Read the model definition and answer for the solid it produces. Units are mm, in the model's axes. A direction names the side the tool comes from. Round coordinates to 2 decimals unless told otherwise and drop trailing zeros. Write each loop counter-clockwise with the first axis right and the second up, starting at its lowest first coordinate (ties: lowest second). Pieces come first, ordered by that corner, then holes. Notation, with made-up numbers: (-6, 45) - (31, 45) arc R25 cw to (31, 80) - close; hole circle Ø2 at (58, 61). An arc over 180 degrees is marked (long way). Use one line per item in the form item = value. Start each with the question number.
1) For a pull along Z with two mould halves and no side action, classify faces 1 (the face through (0, 0, -85)), 2 (the face through (0, 5, 45)), 3 (the face through (-1, 16.07, 47.54)) as released by +Z, released by -Z, zero draft, split by the parting line, or undercut.
2) The part is cut by section B-B, the plane y = -2. Count the separate pieces of the cut face and the enclosed holes in it, plus the area to 3 significant figures.
3) Consider line 1 along Y through (x, z) = (1.6, 61); line 2 along Y through (x, z) = (1.4, -74.5). Determine where each line is inside the solid, lowest interval first. Write a range as from..to.
4) Each of these flat-tipped pins is pushed along its axis until it touches: pin 1 (1.5 mm diameter, centred on x = 0, z = -16.5, fed in from +Y); pin 2 (1.5 mm diameter, centred on x = -0.5, y = 8, fed in from +Z). Where does it stop, or does it pass through?
5) The part is cut by section A-A, the plane z = -29. Give the vertices of the cut face in (x, y), plus the area to 3 significant figures.
6) For faces 4 (the face through (-1, 16.07, -52.46)), 5 (the face through (0, 5, -15)), 6 (the face through (0, 5, 80)), determine the directions among +Z, -Z, +X, -X, +Y, -Y from which every point of the face is accessible in a straight line to the end or side of a thin tool.
from build123d import *

# Parameters (mm, degrees)
SALIENTE_EXTRUIR1_DEPTH = 85
CROQUIS2_W              = 5
CROQUIS2_H              = 25
CORTAR_EXTRUIR1_DEPTH   = 6
CROQUIS3_W              = 5
CROQUIS3_H              = 10
SALIENTE_EXTRUIR2_DEPTH = 45
CROQUIS4_W              = 1
CROQUIS4_H              = 25
CORTAR_EXTRUIR2_DEPTH   = 6


with BuildPart() as part:
    # Croquis1 → Saliente-Extruir1 (new body, symmetric)
    with BuildSketch(Plane.XY):
        with BuildLine():
            Line((-2.5, -17.5), (2.5, -17.5))
            Line((2.5, -17.5), (2.5, 17.5))
            ThreePointArc((2.5, 17.5), (-1.035533906, 16.035533906), (-2.5, 12.5))
            Line((-2.5, 12.5), (-2.5, -17.5))
        make_face()
    extrude(amount=SALIENTE_EXTRUIR1_DEPTH, both=True)

    # Croquis2 → Cortar-Extruir1 (cut, through all)
    with BuildSketch(Plane(origin=(2.5, 0, 0), x_dir=(0, 0, -1), z_dir=(1, 0, 0))):
        with Locations((77.5, 5)):
            Rectangle(CROQUIS2_W, CROQUIS2_H)
        with Locations((67.5, 5)):
            Rectangle(CROQUIS2_W, CROQUIS2_H)
        with Locations((57.5, 5)):
            Rectangle(CROQUIS2_W, CROQUIS2_H)
        with Locations((47.5, 5)):
            Rectangle(CROQUIS2_W, CROQUIS2_H)
        with Locations((37.5, 5)):
            Rectangle(CROQUIS2_W, CROQUIS2_H)
        with Locations((27.5, 5)):
            Rectangle(CROQUIS2_W, CROQUIS2_H)
        with Locations((17.5, 5)):
            Rectangle(CROQUIS2_W, CROQUIS2_H)
        with Locations((7.5, 5)):
            Rectangle(CROQUIS2_W, CROQUIS2_H)
        with Locations((-2.5, 5)):
            Rectangle(CROQUIS2_W, CROQUIS2_H)
        with Locations((-12.5, 5)):
            Rectangle(CROQUIS2_W, CROQUIS2_H)
        with Locations((-22.5, 5)):
            Rectangle(CROQUIS2_W, CROQUIS2_H)
        with Locations((-32.5, 5)):
            Rectangle(CROQUIS2_W, CROQUIS2_H)
        with Locations((-42.5, 5)):
            Rectangle(CROQUIS2_W, CROQUIS2_H)
        with Locations((-52.5, 5)):
            Rectangle(CROQUIS2_W, CROQUIS2_H)
        with Locations((-62.5, 5)):
            Rectangle(CROQUIS2_W, CROQUIS2_H)
        with Locations((-72.5, 5)):
            Rectangle(CROQUIS2_W, CROQUIS2_H)
        with Locations((-82.5, 5)):
            Rectangle(CROQUIS2_W, CROQUIS2_H)
    extrude(amount=-CORTAR_EXTRUIR1_DEPTH, mode=Mode.SUBTRACT)

    # Croquis3 → Saliente-Extruir2 (add)
    with BuildSketch(Plane.XY.offset(85)):
        with Locations((0, -12.5)):
            Rectangle(CROQUIS3_W, CROQUIS3_H)
    extrude(amount=SALIENTE_EXTRUIR2_DEPTH)

    # Croquis4 → Cortar-Extruir2 (cut, through all)
    with BuildSketch(Plane(origin=(2.5, 0, 0), x_dir=(0, 0, -1), z_dir=(1, 0, 0))):
        with Locations((-29.5, 5)):
            Rectangle(CROQUIS4_W, CROQUIS4_H)
        with Locations((30.5, 5)):
            Rectangle(CROQUIS4_W, CROQUIS4_H)
    extrude(amount=-CORTAR_EXTRUIR2_DEPTH, mode=Mode.SUBTRACT)


solid = part.part
Geometry results:
q1.face_1 = released by -Z
q1.face_2 = undercut
q1.face_3 = zero draft
q2.separate_pieces = 17
q2.enclosed_holes = 0
q2.area = 415 mm2
q3.line_1 = -17.5..-7.5
q3.line_2 = -17.5..17.38
q4.pin_1 = -7.5
q4.pin_2 = 80
q5.outline = (-2.5, -17.5) - (2.5, -17.5) - (2.5, -7.5) - (-2.5, -7.5) - close
q5.area = 50.0 mm2
q6.face_4 = +Z, -Z, -X, +Y
q6.face_5 = +X, -X, +Y
q6.face_6 = +Z, +X, -X, +Y
